Check sheet for the modelled part. Datum: model origin and axes. Units: mm. Give positions to 0.01 mm unless a question says otherwise; leave off trailing zeros. Loops run counter-clockwise (first coordinate to the right, second up) from the corner with the lowest first, then second, coordinate; pieces in that order, holes last.
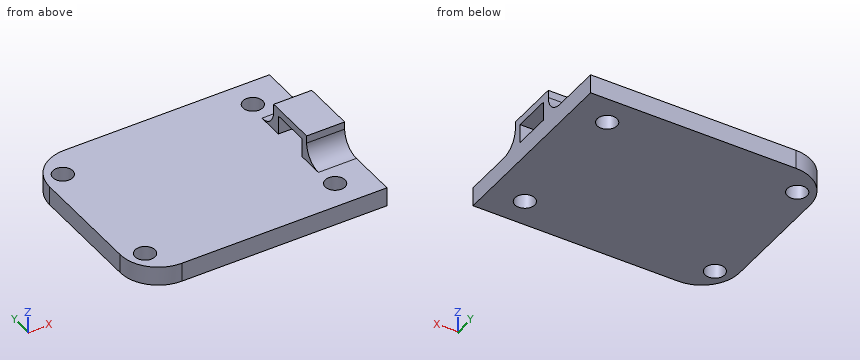
```python
from build123d import *

# Parameters (mm, degrees)
SKETCH1_W           = 64
SKETCH1_H           = 50
SKETCH1_R           = 2.6
BOSS_EXTRUDE1_DEPTH = 5
FILLET1_R           = 10
BOSS_EXTRUDE2_DEPTH = 10
FILLET2_R           = 5


with BuildPart() as part:
    # Sketch1 → Boss-Extrude1 (new body)
    with BuildSketch(Plane.XY):
        with Locations((32, 25)):
            Rectangle(SKETCH1_W, SKETCH1_H)
        with Locations((5, 42.5)):
            Circle(SKETCH1_R, mode=Mode.SUBTRACT)
        with Locations((55, 42.5)):
            Circle(SKETCH1_R, mode=Mode.SUBTRACT)
        with Locations((55, 7.5)):
            Circle(SKETCH1_R, mode=Mode.SUBTRACT)
        with Locations((5, 7.5)):
            Circle(SKETCH1_R, mode=Mode.SUBTRACT)
    extrude(amount=BOSS_EXTRUDE1_DEPTH)

    # Fillet1
    fillet1_edges = [part.edges().sort_by_distance(p)[0] for p in [
        (0, 50, 2.5),
        (0, 0, 2.5),
    ]]
    fillet(fillet1_edges, radius=FILLET1_R)

    # Sketch3 → Boss-Extrude2 (add)
    with BuildSketch(Plane(origin=(64, 0, 0), x_dir=(0, 0, -1), z_dir=(1, 0, 0))):
        Polygon((-5, 30), (-10, 30), (-10, 20), (-5, 20), (-5, 18), (-12, 18), (-12, 32), (-5, 32), align=None)
    extrude(amount=-BOSS_EXTRUDE2_DEPTH)

    # Fillet2
    fillet2_edges = [part.edges().sort_by_distance(p)[0] for p in [
        (59, 32, 5),
        (59, 18, 5),
    ]]
    fillet(fillet2_edges, radius=FILLET2_R)


solid = part.part
```
(1) Gauge pin test, flat ends, axial feed: pin 1 Ø1.6 at (x, z) = (60.5, 11) entering from +Y; pin 2 Ø7 at (x, y) = (5, 7.5) entering from -Z; pin 3 Ø5.5 at (y, z) = (22.5, 9) entering from -X; pin 4 Ø6 at (x, y) = (55, 42.5) entering from +Z. Record the tip position at first contact, or that the pin passes through.
(2) Section check A-A on y = 29. Record the boundary of the cut face in (x, z).
(3) Section check D-D on z = 6. Record the boundary of the cut face in (x, y), plus the area to 3 significant figures.
(4) Section check C-C on z = 2. Record the boundary of the cut face in (x, y), plus the area to 3 significant figures.
(5) Material ranges on line 1 (Y direction, x = 55, z = 1.7); line 2 (Y direction, x = 5, z = 1.3); line 3 (Z direction, x = 24.5, y = 25.5), recorded low to high.
(6) Section check B-B on x = 55. Record the boundary of the cut face in (y, z), plus the area to 3 significant figures.
Computed values:
1. pin 1: stops at y = 32
1. pin 2: stops at z = 0
1. pin 3: stops at x = 54
1. pin 4: stops at z = 5
2. outline: (0, 0) - (64, 0) - (64, 5) - (0, 5) - close; (54, 10) - (64, 10) - (64, 12) - (54, 12) - close
3. outline: (54, 16) - (64, 16) - (64, 20) - (54, 20) - close; (54, 30) - (64, 30) - (64, 34) - (54, 34) - close
3. area: 80.0 mm2
4. outline: (0, 10) arc R10 ccw to (10, 0) - (64, 0) - (64, 50) - (10, 50) arc R10 ccw to (0, 40) - close; hole circle Ø5.2 at (5, 7.5); hole circle Ø5.2 at (5, 42.5); hole circle Ø5.2 at (55, 7.5); hole circle Ø5.2 at (55, 42.5)
4. area: 3,070 mm2
5. line 1: y = 0 to 4.9, 10.1 to 39.9, 45.1 to 50
5. line 2: y = 1.34 to 4.9, 10.1 to 39.9, 45.1 to 48.66
5. line 3: z = 0 to 5
6. outline: (0, 0) - (4.9, 0) - (4.9, 5) - (0, 5) - close; (10.1, 0) - (39.9, 0) - (39.9, 5) - (37, 5) arc R5 cw to (32, 10) - (32, 12) - (18, 12) - (18, 10) arc R5 cw to (13, 5) - (10.1, 5) - close; (45.1, 0) - (50, 0) - (50, 5) - (45.1, 5) - close; hole (20, 5) - (30, 5) - (30, 10) - (20, 10) - close
6. area: 257 mm2
